Check sheet for the modelled part. Datum: model origin and axes. Units: mm. Give positions to 0.01 mm unless a question says otherwise; leave off trailing zeros. Order: outer loops, then holes, each group sorted by start corner. A loop starts at its lowest first (then second) coordinate and runs counter-clockwise, first axis right, second up.
```python
from build123d import *

# Parameters (mm, degrees)
F0_R     = 57.15
F0_R_2   = 6.35
F0_R_3   = 4.7625
F1_DEPTH = 6.35
F2_SIZE  = 0.508
F3_SIZE  = 5.08


# Not quite as in the source:
# - a feature names something its author has since deleted; it is built from what else it names


with BuildPart() as f1:
    # F0 (on Top) → F1 (new body)
    with BuildSketch(Plane.XY):
        Circle(F0_R)
        with Locations((-38.4948291982, -22.225)):
            Circle(F0_R_2, mode=Mode.SUBTRACT)
        with Locations((38.4948291982, -22.225)):
            Circle(F0_R_2, mode=Mode.SUBTRACT)
        Circle(F0_R_3, mode=Mode.SUBTRACT)
        with Locations((0, 44.45)):
            Circle(F0_R_2, mode=Mode.SUBTRACT)
    extrude(amount=F1_DEPTH)

    # F2
    f2_edges = [f1.edges().sort_by_distance(p)[0] for p in [
        (-57.15, 0, 6.35),
        (-6.35, 44.45, 6.35),
        (-44.844829, -22.225, 6.35),
        (32.144829, -22.225, 6.35),
        (-57.15, 0, 0),
        (-6.35, 44.45, 0),
        (32.144829, -22.225, 0),
        (-44.844829, -22.225, 0),
    ]]
    chamfer(f2_edges, length=F2_SIZE)

    # F3
    f3_edges = [f1.edges().sort_by_distance(p)[0] for p in [
        (-4.7625, 0, 0),
    ]]
    chamfer(f3_edges, length=F3_SIZE)


solid = f1.part
```
(1) Material ranges on L1, parallel to Y at x = 0, z = 5.45; L2, parallel to Y at x = 0, z = 5.9; L3, parallel to X at y = -24.5, z = 2.75, recorded low to high.
Response values:
L1: y = -57.15 to -4.76, 4.76 to 38.1, 50.8 to 57.15
L2: y = -57.09 to -4.76, 4.76 to 38.04, 50.86 to 57.09
L3: x = -51.63 to -44.42, -32.57 to 32.57, 44.42 to 51.63
(2) Cross-section at C-C on z = 2.75. Count the separate pieces of the cut face and the enclosed holes in it, then the cut area to 3 significant figures.
Response values:
separate pieces: 1
enclosed holes: 4
area: 9,720 mm2
(3) Release check for a two-part mould opening along X. For faces 1 (the face through (-57.095, 2.513, 3.138)), 2 (the face through (-45, -22, 6)), 3 (the face through (-1, -12, 0)) record: released by +X, released by -X, zero draft, split by the parting line, or undercut.
Response values:
face 1: split by the parting line
face 2: undercut
face 3: zero draft
(4) Cross-section at B-B on x = 0. Enter the section's corners in (y, z).
Response values:
outline: (-57.15, 0.51) - (-56.64, 0) - (-9.84, 0) - (-4.76, 5.08) - (-4.76, 6.35) - (-56.64, 6.35) - (-57.15, 5.84) - close; (4.76, 5.08) - (9.84, 0) - (37.59, 0) - (38.1, 0.51) - (38.1, 5.84) - (37.59, 6.35) - (4.76, 6.35) - close; (50.8, 0.51) - (51.31, 0) - (56.64, 0) - (57.15, 0.51) - (57.15, 5.84) - (56.64, 6.35) - (51.31, 6.35) - (50.8, 5.84) - close
(5) Gauge pin test, flat ends, axial feed: pin 1 Ø2 at (x, z) = (-2.5, 4.5) entering from -Y; pin 2 Ø2 at (y, z) = (26.5, 2) entering from -X. Record the tip position at first contact, or that the pin passes through.
Response values:
pin 1: stops at y = -57.13
pin 2: stops at x = -51.15
(6) Cross-section at A-A on y = 0. Enter the section's corners in (x, z).
Response values:
outline: (-57.15, 0.51) - (-56.64, 0) - (-9.84, 0) - (-4.76, 5.08) - (-4.76, 6.35) - (-56.64, 6.35) - (-57.15, 5.84) - close; (4.76, 5.08) - (9.84, 0) - (56.64, 0) - (57.15, 0.51) - (57.15, 5.84) - (56.64, 6.35) - (4.76, 6.35) - close
